```python
from build123d import *

# Parameters (mm, degrees)
SKETCH_1_R          = 61.5
SKETCH_1_R_2        = 2
SKETCH_1_R_3        = 2.6
SKETCH_1_R_4        = 15.5
EXTRUDE_1_DEPTH     = 2.5
SKETCH_2_R          = 30
CUT_EXTRUDE_1_DEPTH = 10


with BuildPart() as part:
    # 草图1 → 凸台-拉伸1 (new body)
    with BuildSketch(Plane.XY):
        Circle(SKETCH_1_R)
        with Locations((0, -57)):
            Circle(SKETCH_1_R_2, mode=Mode.SUBTRACT)
        with Locations((-40.305086528, -40.305086528)):
            Circle(SKETCH_1_R_2, mode=Mode.SUBTRACT)
        with Locations((-57, 0)):
            Circle(SKETCH_1_R_2, mode=Mode.SUBTRACT)
        with Locations((-40.305086528, 40.305086528)):
            Circle(SKETCH_1_R_2, mode=Mode.SUBTRACT)
        with Locations((0, -23.75)):
            Circle(SKETCH_1_R_3, mode=Mode.SUBTRACT)
        with Locations((-20.56810334, 11.875)):
            Circle(SKETCH_1_R_3, mode=Mode.SUBTRACT)
        with Locations((20.56810334, 11.875)):
            Circle(SKETCH_1_R_3, mode=Mode.SUBTRACT)
        with Locations((19.485571585, -11.25)):
            Circle(SKETCH_1_R_3, mode=Mode.SUBTRACT)
        with Locations((-19.485571585, -11.25)):
            Circle(SKETCH_1_R_3, mode=Mode.SUBTRACT)
        with Locations((0, 22.5)):
            Circle(SKETCH_1_R_3, mode=Mode.SUBTRACT)
        Circle(SKETCH_1_R_4, mode=Mode.SUBTRACT)
        with Locations((0, 57)):
            Circle(SKETCH_1_R_2, mode=Mode.SUBTRACT)
        with Locations((40.305086528, 40.305086528)):
            Circle(SKETCH_1_R_2, mode=Mode.SUBTRACT)
        with Locations((57, 0)):
            Circle(SKETCH_1_R_2, mode=Mode.SUBTRACT)
        with Locations((40.305086528, -40.305086528)):
            Circle(SKETCH_1_R_2, mode=Mode.SUBTRACT)
    extrude(amount=EXTRUDE_1_DEPTH)

    # 草图2 → 切除-拉伸1 (cut)
    with BuildSketch(Plane.XY.offset(2.5)):
        Circle(SKETCH_2_R)
    extrude(amount=-CUT_EXTRUDE_1_DEPTH, mode=Mode.SUBTRACT)


solid = part.part
```
The listing builds one solid part. Answer for the finished solid, in the listing's coordinates (mm). Give positions to 0.01 mm unless a question says otherwise; leave off trailing zeros. Write each loop counter-clockwise with the first axis right and the second up, starting at its lowest first coordinate (ties: lowest second). Pieces come first, ordered by that corner, then holes. Notation, with made-up numbers: (85.25, 78) -> (119.25, 78) arc R26 ccw to (119.25, 98) -> close; hole circle Ø11 at (6.5, -21). An arc over 180 degrees is marked (long way). Write item = value, one per line. Start each with the question number.
1) Straight lines are drawn through the part: line 1 along Y through (x, z) = (0, 0.85); line 2 along Y through (x, z) = (-10, 0.65); line 3 along Y through (x, z) = (-11.5, 1.1). For each, find the intervals that lie inside material, in ascending order.
2) Determine the mould class of faces 1 (the face through (26.5, 14.5, 2.5)), 2 (the face through (42.153, -41.071, 1.232)), 3 (the face through (28.38, -54.56, 1.23)) for opening direction Y: +Y half, -Y half, draft (parallel to the pull), parting line (faces both ways), or undercut.
3) The part is cut by section A-A, the plane x = 0. Determine the outline of the cut face in (y, z).
4) The part is cut by section D-D, the plane y = 57. Determine the outline of the cut face in (x, z).
5) The part is cut by section C-C, the plane x = -26.5. Determine the outline of the cut face in (y, z), and give its area (3 significant figures).
Solutions:
q1.line_1 = -61.5 to -59, -55 to -30, 30 to 55, 59 to 61.5
q1.line_2 = -60.68 to -28.28, 28.28 to 60.68
q1.line_3 = -60.42 to -27.71, 27.71 to 60.42
q2.face_1 = draft
q2.face_2 = undercut
q2.face_3 = parting line
q3.outline = (-61.5, 0) -> (-59, 0) -> (-59, 2.5) -> (-61.5, 2.5) -> close; (-55, 0) -> (-30, 0) -> (-30, 2.5) -> (-55, 2.5) -> close; (30, 0) -> (55, 0) -> (55, 2.5) -> (30, 2.5) -> close; (59, 0) -> (61.5, 0) -> (61.5, 2.5) -> (59, 2.5) -> close
q4.outline = (-23.09, 0) -> (-2, 0) -> (-2, 2.5) -> (-23.09, 2.5) -> close; (2, 0) -> (23.09, 0) -> (23.09, 2.5) -> (2, 2.5) -> close
q5.outline = (-55.5, 0) -> (-14.06, 0) -> (-14.06, 2.5) -> (-55.5, 2.5) -> close; (14.06, 0) -> (55.5, 0) -> (55.5, 2.5) -> (14.06, 2.5) -> close
q5.area = 207 mm²
